Part model, mm, in its own coordinate system. A direction names the side the tool comes from. Round coordinates to 2 decimals unless told otherwise and drop trailing zeros. Loops run counter-clockwise (first coordinate to the right, second up) from the corner with the lowest first, then second, coordinate; pieces in that order, holes last. Notation, with made-up numbers: (-19, 8) - (26, 8) arc R22 ccw to (26, 27) - close; hole circle Ø6 at (88.5, 33). An arc over 180 degrees is marked (long way). Put each result on its own line as item: value.
from build123d import *

# Parameters (mm, degrees)
F1_DEPTH     = 88.9
F2_T1_DEPTH  = 88.9
F2_T3_DEPTH  = 88.9
F2_T5_DEPTH  = 149.5881510316
F2_T7_DEPTH  = 114.3
F2_T9_DEPTH  = 33.3375
F2_T11_DEPTH = 33.3375
F2_T13_DEPTH = 114.3


# Not quite as in the source:
# - a fillet or chamfer that OpenCascade refuses, or shapes differently, is made with other operations: its cross-section is extruded or revolved along the edge and cut away or added


with BuildPart() as f1:
    # F0 (on Right) → F1 (new body)
    with BuildSketch(Plane.YZ):
        Polygon((-11.2253201513, 0), (0, 0), (-101.027881362, 101.027881362), (-190.8304425727, 11.2253201513), (-204.3008267543, 24.6957043329), (-209.91348683, 19.0830442573), (-190.8304425727, 0), (-101.027881362, 89.8025612107), align=None)
    extrude(amount=-F1_DEPTH)

    # F2: fillet of radius 5.08 on 7 edges, made by hand

    # F2_s2 → F2_t1 (join)
    with BuildSketch(Plane.YZ.offset(-88.9)):
        with BuildLine():
            ThreePointArc((-97.4357789136, 86.2104587623), (-101.027881362, 87.6983563138), (-104.6199838105, 86.2104587623))
            Line((-104.6199838105, 86.2104587623), (-101.027881362, 89.8025612107))
            Line((-101.027881362, 89.8025612107), (-97.4357789136, 86.2104587623))
        make_face()
    extrude(amount=F2_T1_DEPTH)

    # F2_s4 → F2_t3 (join)
    with BuildSketch(Plane.YZ.offset(-88.9)):
        with BuildLine():
            ThreePointArc((-187.2383401243, 14.8174225998), (-190.8304425727, 13.3295250482), (-194.4225450211, 14.8174225998))
            Line((-194.4225450211, 14.8174225998), (-190.8304425727, 11.2253201513))
            Line((-190.8304425727, 11.2253201513), (-187.2383401243, 14.8174225998))
        make_face()
    extrude(amount=F2_T3_DEPTH)

    # F2_s6 → F2_t5 (cut)
    with BuildSketch(Plane.YZ.offset(-119.2440755158)):
        with BuildLine():
            ThreePointArc((-11.2253201513, 0), (-7.3196509923, 3.4955502605), (-8.5826006264, 8.5826006264))
            Line((-8.5826006264, 8.5826006264), (0, 0))
            Line((0, 0), (-11.2253201513, 0))
        make_face()
    extrude(amount=F2_T5_DEPTH, mode=Mode.SUBTRACT)

    # F2_s8 → F2_t7 (cut)
    with BuildSketch(Plane.YZ.offset(-101.6)):
        with BuildLine():
            ThreePointArc((-104.6199838105, 97.4357789136), (-101.027881362, 98.9236764652), (-97.4357789136, 97.4357789136))
            Line((-97.4357789136, 97.4357789136), (-101.027881362, 101.027881362))
            Line((-101.027881362, 101.027881362), (-104.6199838105, 97.4357789136))
        make_face()
    extrude(amount=F2_T7_DEPTH, mode=Mode.SUBTRACT)

    # F2_s10 → F2_t9 (cut)
    with BuildSketch(Plane(origin=(0, -80.8223050896, -80.8223050896), x_dir=(1, 0, 0), z_dir=(0, -0.7071067812, -0.7071067812))):
        with BuildLine():
            ThreePointArc((0, 156.845), (-1.4878975516, 160.4371024484), (-5.08, 161.925))
            Line((-5.08, 161.925), (0, 161.925))
            Line((0, 161.925), (0, 156.845))
        make_face()
    extrude(amount=F2_T9_DEPTH, mode=Mode.SUBTRACT)

    # F2_s12 → F2_t11 (cut)
    with BuildSketch(Plane(origin=(0, -80.8223050896, -80.8223050896), x_dir=(1, 0, 0), z_dir=(0, -0.7071067812, -0.7071067812))):
        with BuildLine():
            ThreePointArc((-88.9, 156.845), (-87.4121024484, 160.4371024484), (-83.82, 161.925))
            Line((-83.82, 161.925), (-88.9, 161.925))
            Line((-88.9, 161.925), (-88.9, 156.845))
        make_face()
    extrude(amount=F2_T11_DEPTH, mode=Mode.SUBTRACT)

    # F2_s14 → F2_t13 (cut)
    with BuildSketch(Plane.YZ.offset(-101.6)):
        with BuildLine():
            ThreePointArc((-187.2383401243, 3.5921024484), (-190.8304425727, 2.1042048969), (-194.4225450211, 3.5921024484))
            Line((-194.4225450211, 3.5921024484), (-190.8304425727, 0))
            Line((-190.8304425727, 0), (-187.2383401243, 3.5921024484))
        make_face()
    extrude(amount=F2_T13_DEPTH, mode=Mode.SUBTRACT)


solid = f1.part
1. Probe line 1 along Y through (x, z) = (-41, 18); line 2 along Y through (x, z) = (-39.5, 73); line 3 along Y through (x, z) = (-29, 46.5). List the from-to ranges inside material, lowest first. Write a range as [from, to].
A:
line 1: y = [-208.83, -197.61], [-184.06, -172.83], [-29.23, -18]
line 2: y = [-129.06, -117.83], [-84.23, -73]
line 3: y = [-155.56, -144.33], [-57.73, -46.5]
2. Pin check, flat tips, straight feed: P1, Ø1, axis at x = -20.5, z = 61.5, coming from the -Y side; P2, Ø8, axis at x = -44, z = 86, coming from the +Y side; P3, Ø10, axis at x = -68, y = -89.5, coming from the +Z side. Stop position of each tip, or through.
A:
P1: stops at y = -141.06
P2: stops at y = -82
P3: stops at z = 94.5
3. Tool access for faces 1 (the flat face through (-43.83, -202.28, 11.45)), 2 (the flat face through (-43.828, -199.293, 19.687)), 3 (the flat face through (-43.83, -146.51, 44.32)): list every direction of +Z, -Z, +X, -X, +Y, -Y with a clear straight run to the whole face (end or side of a thin tool).
A:
face 1: -Z, +X, -X, -Y
face 2: +Z, +X, -X
face 3: -Z, +X, -X
4. Band-saw the part on B-B (z = 29). List the corners of the cut face in (x, y), plus the area to 3 significant figures.
A:
outline: (-88.9, -173.06) - (0, -173.06) - (0, -161.83) - (-88.9, -161.83) - close; (-88.9, -40.23) - (0, -40.23) - (0, -29) - (-88.9, -29) - close
area: 2,000 mm²
5. Band-saw the part on A-A (x = -36.5). List the corners of the cut face in (y, z).
A:
outline: (-209.91, 19.08) - (-194.42, 3.59) arc R5.08 ccw to (-187.24, 3.59) - (-104.62, 86.21) arc R5.08 cw to (-97.44, 86.21) - (-11.23, 0) arc R5.08 ccw to (-8.58, 8.58) - (-97.44, 97.44) arc R5.08 ccw to (-104.62, 97.44) - (-187.24, 14.82) arc R5.08 cw to (-194.42, 14.82) - (-204.3, 24.7) - close
6. Band-saw the part on C-C (y = -130). List the corners of the cut face in (x, z).
A:
outline: (-88.9, 60.83) - (0, 60.83) - (0, 72.06) - (-88.9, 72.06) - close
7. Two-plate mould, pull along Y, no slides. Class faces 4 (the flat face through (-43.828, -54.934, 43.709)), 5 (the cylindrical face through (-87.45, -205.99, 20.85)), 6 (the flat face through (-88.9, -129, 64)): pulls with the +Y half, pulls with the -Y half, needs draft (parallel to the pull), parting line crosses it, or undercut.
A:
face 4: undercut
face 5: pulls with the -Y half
face 6: needs draft
